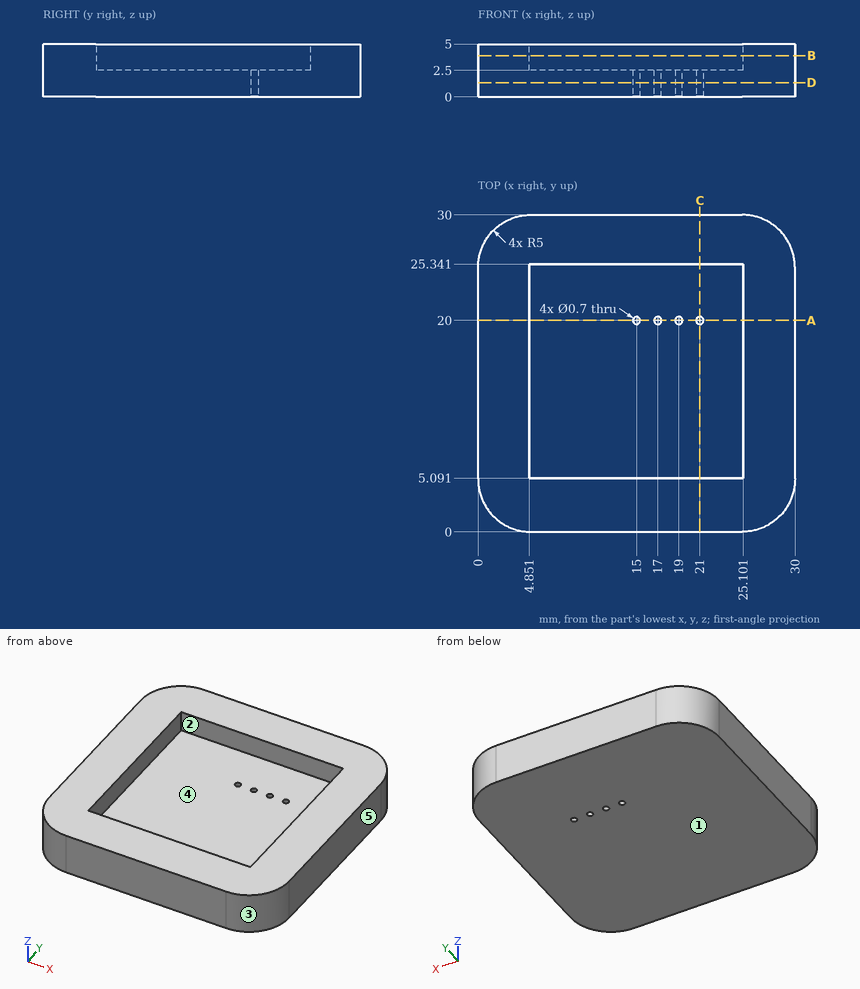
Geometry: see drawing. Coordinates: mm, zero at the bounding-box minimum. A direction names the side the tool comes from. Coordinates: 2 decimals unless noted, no trailing zeros. Order: outer loops, then holes, each group sorted by start corner. A loop starts at its lowest first (then second) coordinate and runs counter-clockwise, first axis right, second up. Notation, with made-up numbers: (-12.5, 35.25) - (8.5, 35.25) arc R23 cw to (8.5, 72.25) - close; hole circle Ø7 at (1.5, 63.25). An arc over 180 degrees is marked (long way). Write each question's results on one line, items separated by ' | '.
1) Section B-B, the plane z = 3.9. Return loops of the section in (x, y).
Results list:
outline: (0, 5) arc R5 ccw to (5, 0) - (25, 0) arc R5 ccw to (30, 5) - (30, 25) arc R5 ccw to (25, 30) - (5, 30) arc R5 ccw to (0, 25) - close; hole (4.85, 5.09) - (25.1, 5.09) - (25.1, 25.34) - (4.85, 25.34) - close
2) Section D-D, the plane z = 1.35. Return loops of the section in (x, y).
Results list:
outline: (0, 5) arc R5 ccw to (5, 0) - (25, 0) arc R5 ccw to (30, 5) - (30, 25) arc R5 ccw to (25, 30) - (5, 30) arc R5 ccw to (0, 25) - close; hole circle Ø0.7 at (15, 20); hole circle Ø0.7 at (17, 20); hole circle Ø0.7 at (19, 20); hole circle Ø0.7 at (21, 20)
3) Section C-C, the plane x = 21. Return loops of the section in (y, z).
Results list:
outline: (0, 0) - (19.65, 0) - (19.65, 2.5) - (5.09, 2.5) - (5.09, 5) - (0, 5) - close; (20.35, 0) - (30, 0) - (30, 5) - (25.34, 5) - (25.34, 2.5) - (20.35, 2.5) - close
4) Set-up query: the marked faces 4 and 5. Return all of +Z, -Z, +X, -X, +Y, -Y with unobstructed straight access to the full face (end or side cutting, diameter ignored); none if empty.
Results list:
face 4: +Z | face 5: +Z, -Z, +X, +Y, -Y
5) Line query: line 1 (X direction, y = 20, z = 1); line 2 (Y direction, x = 21.25, z = 3.95); line 3 (Y direction, x = 15, z = 0.75). Output: solid intervals per line, ascending. Write a range as from..to.
Results list:
line 1: 0..14.65, 15.35..16.65, 17.35..18.65, 19.35..20.65, 21.35..30 | line 2: 0..5.09, 25.34..30 | line 3: 0..19.65, 20.35..30
6) Pull-direction query (X, two-part tool) for the marked faces 1, 2 and 3; classes: pulls with the +X half, pulls with the -X half, needs draft (parallel to the pull), parting line crosses it, or undercut.
Results list:
face 1: needs draft | face 2: undercut | face 3: pulls with the +X half
7) Section A-A, the plane y = 20. Return loops of the section in (x, z).
Results list:
outline: (0, 0) - (14.65, 0) - (14.65, 2.5) - (4.85, 2.5) - (4.85, 5) - (0, 5) - close; (15.35, 0) - (16.65, 0) - (16.65, 2.5) - (15.35, 2.5) - close; (17.35, 0) - (18.65, 0) - (18.65, 2.5) - (17.35, 2.5) - close; (19.35, 0) - (20.65, 0) - (20.65, 2.5) - (19.35, 2.5) - close; (21.35, 0) - (30, 0) - (30, 5) - (25.1, 5) - (25.1, 2.5) - (21.35, 2.5) - close
